Check sheet for the modelled part. Datum: model origin and axes. Units: mm. A direction names the side the tool comes from. Give positions to 0.01 mm unless a question says otherwise; leave off trailing zeros. Loops run counter-clockwise (first coordinate to the right, second up) from the corner with the lowest first, then second, coordinate; pieces in that order, holes last. Notation, with made-up numbers: M -9,84 L 20,84 A12 ccw 20,89 Z; hole C -29.75,5 d5. An arc over 180 degrees is marked long. Use one line per item in the form item = value.
Autodesk Inventor part; units mm, degrees
ref_plane "YZ Plane" through (0, 0, 0) normal (1, 0, 0) x (0, 1, 0)
ref_plane "XZ Plane" through (0, 0, 0) normal (0, 1, 0) x (-1, 0, 0)
ref_plane "XY Plane" through (0, 0, 0) normal (0, 0, 1) x (1, 0, 0)
sketch "スケッチ1" plane through (0, 0, 0) normal (0, 1, 0) x (-1, 0, 0)
  line L0 (-25, -16.9) -> (25, -16.9)
  line L1 (25, -16.9) -> (25, 25)
  line L2 (25, 25) -> (-25, 25)
  line L3 (-25, 25) -> (-25, -16.9)
  point P0 (0, 0)
  point P1 (0, 25)
  dimension "d0" = 50
  dimension "d62" = 25
  dimension "d63" = 16.9
extrude "押し出し1" add sketch "スケッチ1" along normal blind 5
sketch "スケッチ2" plane through (0, 5, 0) normal (0, 1, 0) x (1, 0, 0)
  circle A0 centre (0, 0) radius 16.5
  dimension "d4" = 33
extrude "押し出し2" cut sketch "スケッチ2" against normal blind 5
sketch "スケッチ3" plane through (0, 5, 0) normal (0, 1, 0) x (1, 0, 0)
  line L0 (-6, -17.5) -> (6, -17.5)
  line L1 (6, -17.5) -> (6, -20.5)
  line L2 (6, -20.5) -> (-6, -20.5)
  line L3 (-6, -20.5) -> (-6, -17.5)
  line L4 (-6, -17.5) -> (6, -20.5) construction
  line L5 (6, -17.5) -> (-6, -20.5) construction
  line L6 (-14.7535, 15.4462) -> (-20.7535, 5.0538)
  line L7 (-20.7535, 5.0538) -> (-18.1554, 3.5538)
  line L8 (-18.1554, 3.5538) -> (-12.1554, 13.9462)
  line L9 (-12.1554, 13.9462) -> (-14.7535, 15.4462)
  line L10 (-14.7535, 15.4462) -> (-18.1554, 3.5538) construction
  line L11 (-20.7535, 5.0538) -> (-12.1554, 13.9462) construction
  line L12 (-25, 16.9) -> (-25, -25)
  line L13 (12.1554, 13.9462) -> (18.1554, 3.5538)
  line L14 (18.1554, 3.5538) -> (20.7535, 5.0538)
  line L15 (20.7535, 5.0538) -> (14.7535, 15.4462)
  line L16 (14.7535, 15.4462) -> (12.1554, 13.9462)
  line L17 (12.1554, 13.9462) -> (20.7535, 5.0538) construction
  line L18 (18.1554, 3.5538) -> (14.7535, 15.4462) construction
  line L19 (25, -25) -> (25, 16.9)
  point P0 (0, 0)
  point P1 (0, -19)
  point P2 (-16.4545, 9.5)
  point P3 (16.4545, 9.5)
  point P4 (16.4545, 9.5)
  point P5 (16.4545, 9.5)
  dimension "d7" = 120
  dimension "d8" = 120
  dimension "d9" = 19
  dimension "d10" = 19
  dimension "d11" = 19
  dimension "d12" = 3
  dimension "d13" = 12
  dimension "d14" = 30
  dimension "d15" = 12
  dimension "d16" = 3
  dimension "d17" = 30
  dimension "d18" = 3
  dimension "d19" = 12
extrude "押し出し3" cut sketch "スケッチ3" against normal blind 3
sketch "スケッチ4" plane through (0, 5, 0) normal (0, 1, 0) x (1, 0, 0)
  line L0 (2.5, -15.25) -> (2.5, -22.75)
  line L1 (2.5, -22.75) -> (-2.5, -22.75)
  line L2 (-2.5, -22.75) -> (-2.5, -15.25)
  line L3 (-2.5, -15.25) -> (2.5, -15.25)
  line L4 (2.5, -15.25) -> (-2.5, -22.75) construction
  line L5 (2.5, -22.75) -> (-2.5, -15.25) construction
  line L6 (18.4521, 13.5401) -> (11.9569, 9.7901)
  line L7 (11.9569, 9.7901) -> (14.4569, 5.4599)
  line L8 (14.4569, 5.4599) -> (20.9521, 9.2099)
  line L9 (20.9521, 9.2099) -> (18.4521, 13.5401)
  line L10 (18.4521, 13.5401) -> (14.4569, 5.4599) construction
  line L11 (11.9569, 9.7901) -> (20.9521, 9.2099) construction
  line L12 (25, -25) -> (25, 16.9)
  line L13 (-18.4521, 13.5401) -> (-11.9569, 9.7901)
  line L14 (-11.9569, 9.7901) -> (-14.4569, 5.4599)
  line L15 (-14.4569, 5.4599) -> (-20.9521, 9.2099)
  line L16 (-20.9521, 9.2099) -> (-18.4521, 13.5401)
  line L17 (-18.4521, 13.5401) -> (-14.4569, 5.4599) construction
  line L18 (-11.9569, 9.7901) -> (-20.9521, 9.2099) construction
  line L19 (-25, 16.9) -> (-25, -25)
  point P0 (0, 0)
  point P1 (16.4545, 9.5)
  point P2 (0, -19)
  point P3 (-16.4545, 9.5)
  dimension "d28" = 120
  dimension "d29" = 120
  dimension "d30" = 19
  dimension "d31" = 19
  dimension "d32" = 19
  dimension "d33" = 30
  dimension "d34" = 7.5
  dimension "d35" = 5
  dimension "d38" = 7.5
  dimension "d39" = 5
  dimension "d40" = 5
  dimension "d41" = 7.5
  dimension "d42" = 30
extrude "押し出し4" cut sketch "スケッチ4" against normal blind 5
sketch "スケッチ5" plane through (0, 5, 0) normal (0, 1, 0) x (1, 0, 0)
  line L0 (-25, -25) -> (25, -25)
  line L1 (25, 16.9) -> (-25, 16.9)
  line L2 (-25, 16.9) -> (-25, -25)
  line L3 (25, -25) -> (25, 16.9)
  point P0 (0, 0)
  point P1 (21, -20)
  point P2 (-21, -20)
  point P3 (-21, 0)
  point P4 (21, 0)
  point P5 (15, 0)
  point P6 (-15, 0)
  dimension "d45" = 5
  dimension "d48" = 5
  dimension "d49" = 4
  dimension "d50" = 4
  dimension "d51" = 4
  dimension "d52" = 4
  dimension "d60" = 6
  dimension "d61" = 6
  dimension "d64" = 20
hole "穴1" at (21, 5, 20) at (-21, 5, 20) at (-21, 5, 0) at (21, 5, 0) at (15, 5, 0) at (-15, 5, 0) direction (0, -1, 0) diameter 3 end through all
properties part number "trackball_base" material "アルミニウム 6061"
1) Set-up check for faces 1 (the face through (19.436, 3.521, -4.293)), 2 (the face through (19.72, 2.54, -11.34)), 3 (the face through (25, 2, 4)): record each of +Z, -Z, +X, -X, +Y, -Y from which the full face is reachable in a straight line by a thin tool's end or side.
Evaluation:
face_1 = +Y
face_2 = +Y, -Y
face_3 = +Z, -Z, +X, +Y, -Y
2) Section check C-C (y = 1.2). Record the cut outline in (x, z).
Evaluation:
outline = M -25,-16.9 L 25,-16.9 L 25,25 L -25,25 Z; hole C -21,0 d3; hole C -21,20 d3; hole M -20.95,-9.21 L -18.45,-13.54 L -12.87,-10.32 A16.5 ccw 12.87,-10.32 L 18.45,-13.54 L 20.95,-9.21 L 15.37,-5.99 A16.5 ccw 2.5,16.31 L 2.5,22.75 L -2.5,22.75 L -2.5,16.31 A16.5 ccw -15.37,-5.99 Z; hole C 21,0 d3; hole C 21,20 d3
3) Release check for a two-part mould opening along Z. For faces 4 (the face through (0, 2, -16.9)), 5 (the face through (6, 0, 18)), 6 (the face through (17.27, 3.52, -5.09)) record: pulls with the +Z half, pulls with the -Z half, needs draft (parallel to the pull), parting line crosses it, or undercut.
Evaluation:
face_4 = pulls with the -Z half
face_5 = needs draft
face_6 = undercut
4) Section check D-D (z = 15.5). Record the cut outline in (x, y).
Evaluation:
outline = M -25,0 L -5.66,0 L -5.66,5 L -25,5 Z; M 5.66,0 L 25,0 L 25,5 L 5.66,5 Z
5) Section check B-B (x = 8). Record the cut outline in (y, z).
Evaluation:
outline = M 0,-16.9 L 5,-16.9 L 5,-14.43 L 0,-14.43 Z; M 0,14.43 L 5,14.43 L 5,25 L 0,25 Z
6) Section check A-A (z = 0). Record the cut outline in (x, y), then the cut area to 3 significant figures.
Evaluation:
outline = M -25,0 L -22.5,0 L -22.5,5 L -25,5 Z; M -19.5,0 L -16.5,0 L -16.5,5 L -19.5,5 Z; M 16.5,0 L 19.5,0 L 19.5,5 L 16.5,5 Z; M 22.5,0 L 25,0 L 25,5 L 22.5,5 Z
area = 55.0 mm^2
7) Depth check by flat-ended pin: pin 1 Ø1.3 at (x, z) = (-14.5, -13.5) entering from +Y. Enter the tip coordinate at first touch or a pass-through.
Evaluation:
pin_1 = 2
8) Scan lines: line 1 (X direction, y = 1.85, z = 20); line 2 (X direction, y = 1.75, z = 0); line 3 (Z direction, x = -21, y = 1.4). Record each from-to range of solid material in increasing order.
Evaluation:
line_1 = -25 to -22.5, -19.5 to -2.5, 2.5 to 19.5, 22.5 to 25
line_2 = -25 to -22.5, -19.5 to -16.5, 16.5 to 19.5, 22.5 to 25
line_3 = -16.9 to -1.5, 1.5 to 18.5, 21.5 to 25
